from build123d import *

# Parameters (mm, degrees)
F1_DEPTH = 25.4
F3_DEPTH = 25.4
F4_R     = 5.457243
F5_DEPTH = 25.4
F6_R     = 6.556399
F7_DEPTH = 12.7
F8_R     = 6.526479
F9_DEPTH = 25.4


with BuildPart() as f1:
    # F0 (on Front) → F1 (new body)
    with BuildSketch(Plane.XZ):
        Polygon((-13.941352, 12.7), (-13.941352, 0), (62.258648, 0), (62.258648, 12.7), (36.858648, 12.7), (36.858648, 44.45), (11.458648, 44.45), (11.458648, 12.7), align=None)
    extrude(amount=F1_DEPTH)

    # F2 (on face) → F3 (cut)
    with BuildSketch(Plane.YZ.offset(36.858648)):
        with BuildLine():
            ThreePointArc((-25.4, 33.849411), (-20.7886, 41.232629), (-12.7, 44.45))
            Line((-12.7, 44.45), (-25.4, 44.45))
            Line((-25.4, 44.45), (-25.4, 33.849411))
        make_face()
        with BuildLine():
            Line((0, 44.45), (-12.7, 44.45))
            ThreePointArc((-12.7, 44.45), (-4.617872, 41.224876), (0, 33.849411))
            Line((0, 33.849411), (0, 44.45))
        make_face()
    extrude(amount=-F3_DEPTH, mode=Mode.SUBTRACT)

    # F4 (on face) → F5 (cut)
    with BuildSketch(Plane.YZ.offset(36.858648)):
        with Locations((-12.7, 36.11993)):
            Circle(F4_R)
    extrude(amount=-F5_DEPTH, mode=Mode.SUBTRACT)

    # F6 (on face) → F7 (cut)
    with BuildSketch(Plane.XY.offset(12.7)):
        with BuildLine():
            Line((-13.941352, 0), (-13.941352, -12.7))
            ThreePointArc((-13.941352, -12.7), (-10.016193, -3.925159), (-1.241352, 0))
            Line((-1.241352, 0), (-13.941352, 0))
        make_face()
        with BuildLine():
            ThreePointArc((-1.241352, -25.4), (-9.966637, -21.425286), (-13.941352, -12.7))
            Line((-13.941352, -12.7), (-13.941352, -25.4))
            Line((-13.941352, -25.4), (-1.241352, -25.4))
        make_face()
        with Locations((-2.420933, -12.7)):
            Circle(F6_R)
    extrude(amount=-F7_DEPTH, mode=Mode.SUBTRACT)

    # F8 (on face) → F9 (cut)
    with BuildSketch(Plane.XY.offset(12.7)):
        with Locations((50.674323, -12.7)):
            Circle(F8_R)
        with BuildLine():
            ThreePointArc((49.558648, 0), (58.40559, -3.853059), (62.258648, -12.7))
            Line((62.258648, -12.7), (62.258648, 0))
            Line((62.258648, 0), (49.558648, 0))
        make_face()
        with BuildLine():
            Line((62.258648, -25.4), (62.258648, -12.7))
            ThreePointArc((62.258648, -12.7), (58.437118, -21.57847), (49.558648, -25.4))
            Line((49.558648, -25.4), (62.258648, -25.4))
        make_face()
    extrude(amount=-F9_DEPTH, mode=Mode.SUBTRACT)


solid = f1.part
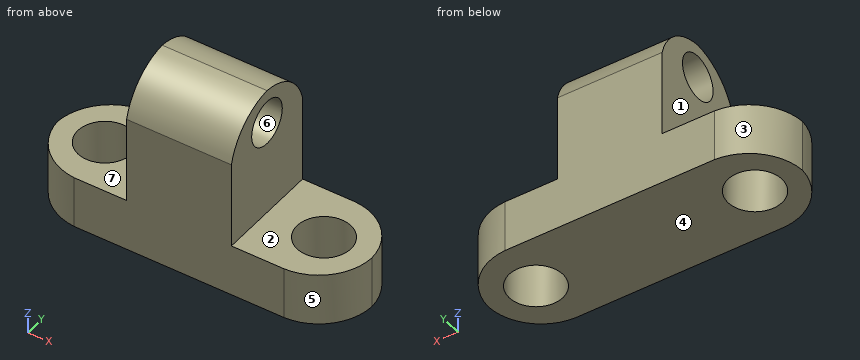
Here's how the part is built. I have some questions about the finished solid (model axes, mm). Face numbers are marked on the shaded views. A direction names the side the tool comes from. Give positions to 0.01 mm unless a question says otherwise; leave off trailing zeros. Order: outer loops, then holes, each group sorted by start corner. A loop starts at its lowest first (then second) coordinate and runs counter-clockwise, first axis right, second up. Notation, with made-up numbers: (78.5, 22.5) -> (125.5, 22.5) arc R13 ccw to (125.5, 31.5) -> close; hole circle Ø1 at (4.5, -9.5). An arc over 180 degrees is marked (long way). One line per item, written item: value. Start each with the question number.
1. Imagine slicing it at A-A, the plane y = -9.75. List the corners of the cut face in (x, z) for me, plus the area to 3 significant figures.
2. We'd pull the mould along Z, two halves only. Please class the marked faces 4, 5, 6 and 7: released by +Z, released by -Z, zero draft, split by the parting line, or undercut.
3. Imagine slicing it at C-C, the plane x = 15. List the corners of the cut face in (y, z) for me.
4. Imagine slicing it at D-D, the plane z = 20.5. List the corners of the cut face in (x, y) for me, plus the area to 3 significant figures.
5. Imagine slicing it at B-B, the plane z = 9.5. List the corners of the cut face in (x, y) for me, plus the area to 3 significant figures.
6. I need wall thicknesses on probe 1 along Z at (x, y) = (19, -12.7); probe 2 along X at (y, z) = (-21.25, 39); probe 3 along Z at (x, y) = (2, -5). Which ranges of each line are inside material? Lowest first, please. Write a range as from..to.
7. For the marked faces 1, 2 and 3, which set-ups out of +Z, -Z, +X, -X, +Y, -Y let a thin tool reach every point of the face, with its end or its side?
8. Will these pins go through, and if not, where does the flat tip stop? pin 1 Ø1 at (x, y) = (47, -22) entering from +Z; pin 2 Ø12 at (x, y) = (-2.42, -12.7) entering from -Z; pin 3 Ø2 at (y, z) = (-6.5, 21) entering from +X; pin 4 Ø6 at (y, z) = (-20.5, 14.5) entering from -X.
Values follow:
1. outline: (-13.44, 0) -> (-8.28, 0) -> (-8.28, 12.7) -> (-13.44, 12.7) -> close; (3.43, 0) -> (44.85, 0) -> (44.85, 12.7) -> (36.86, 12.7) -> (36.86, 31.53) -> (11.46, 31.53) -> (11.46, 12.7) -> (3.43, 12.7) -> close; (11.46, 40.71) -> (36.86, 40.71) -> (36.86, 43.94) -> (11.46, 43.94) -> close; (56.5, 0) -> (61.81, 0) -> (61.81, 12.7) -> (56.5, 12.7) -> close
1. area: 1,220 mm2
2. face 4: released by -Z
2. face 5: zero draft
2. face 6: undercut
2. face 7: released by +Z
3. outline: (-25.4, 0) -> (0, 0) -> (0, 33.85) arc R14.01 ccw to (-12.7, 44.45) arc R13.96 ccw to (-25.4, 33.85) -> close; hole circle Ø10.91 at (-12.7, 36.12)
4. outline: (11.46, -25.4) -> (36.86, -25.4) -> (36.86, 0) -> (11.46, 0) -> close
4. area: 645 mm2
5. outline: (-13.94, -12.7) arc R13.68 ccw to (-1.24, -25.4) -> (49.56, -25.4) arc R13.06 ccw to (62.26, -12.7) arc R13.18 ccw to (49.56, 0) -> (-1.24, 0) arc R13.47 ccw to start; hole circle Ø13.11 at (-2.42, -12.7); hole circle Ø13.05 at (50.67, -12.7)
5. area: 1,520 mm2
6. probe 1: z = 0..30.66, 41.58..44.45
6. probe 2: x = 11.46..36.86
6. probe 3: z = 0..12.7
7. face 1: +Z, -X, +Y, -Y
7. face 2: +Z, +X, +Y, -Y
7. face 3: +Z, -Z, -X, +Y
8. pin 1: stops at z = 12.7
8. pin 2: passes through
8. pin 3: stops at x = 36.86
8. pin 4: stops at x = -12.41
